For this review, take the finished solid that the model builds, in its own axes (mm). A direction names the side the tool comes from. Coordinates: 2 decimals unless noted, no trailing zeros. Write each loop counter-clockwise with the first axis right and the second up, starting at its lowest first coordinate (ties: lowest second). Pieces come first, ordered by that corner, then holes. Notation, with made-up numbers: M 8,76 L 25,76 A12 cw 25,91 Z; hole C -6,63 d9. An arc over 180 degrees is marked long. Return JSON: item names as keys, results as strings.
```python
from build123d import *

# Parameters (mm, degrees)
SKETCH2_R            = 9.9
BOSS_EXTRUDE1_DEPTH  = 1.225
SKETCH3_R            = 4.5
BOSS_EXTRUDE2_DEPTH  = 2.05
M3_CLEARANCE_HOLE1_D = 3.4


with BuildPart() as part:
    # Sketch2 → Boss-Extrude1 (new body, symmetric)
    with BuildSketch(Plane(origin=(0, 0, 0), x_dir=(1, 0, 0), z_dir=(0, 1, 0))):
        Circle(SKETCH2_R)
    extrude(amount=BOSS_EXTRUDE1_DEPTH, both=True)

    # Sketch3 → Boss-Extrude2 (add)
    with BuildSketch(Plane(origin=(0, 1.225, 0), x_dir=(1, 0, 0), z_dir=(0, 1, 0))):
        Circle(SKETCH3_R)
    extrude(amount=BOSS_EXTRUDE2_DEPTH)

    # M3 Clearance Hole1 (through all)
    with Locations(Plane(origin=(0, -1.225, 0), x_dir=(-1, 0, 0), z_dir=(0, -1, 0))):
        with Locations((0, 0), (0, 7), (7, 0), (0, -7), (-7, 0)):
            Hole(M3_CLEARANCE_HOLE1_D / 2)


solid = part.part
```
1. We need section C-C (x = 6). State the section outline as (y, z) points (3 decimals).
Checks:
{"outline": "M -1.225,-7.875 L 1.225,-7.875 L 1.225,-1.375 L -1.225,-1.375 Z; M -1.225,1.375 L 1.225,1.375 L 1.225,7.875 L -1.225,7.875 Z"}
2. Clearance check with flat-ended pins moving along their axes: pin 1 Ø1 at (y, z) = (1.5, 6.5) entering from +X; pin 2 Ø1.5 at (x, y) = (3, 1) entering from +Z; pin 3 Ø1 at (x, z) = (-6.5, -5) entering from +Y (3 decimals). State where each tip first meets the part, or that it passes through.
Checks:
{"pin 1": "x = 7.81", "pin 2": "z = 9.64", "pin 3": "y = 1.225"}
3. We need section A-A (z = 0). State the section outline as (x, y) points (3 decimals), plus the area to 3 significant figures.
Checks:
{"outline": "M -9.9,-1.225 L -8.7,-1.225 L -8.7,1.225 L -9.9,1.225 Z; M -5.3,-1.225 L -1.7,-1.225 L -1.7,3.275 L -4.5,3.275 L -4.5,1.225 L -5.3,1.225 Z; M 1.7,-1.225 L 5.3,-1.225 L 5.3,1.225 L 4.5,1.225 L 4.5,3.275 L 1.7,3.275 Z; M 8.7,-1.225 L 9.9,-1.225 L 9.9,1.225 L 8.7,1.225 Z", "area": "35.0 mm2"}
4. We need section B-B (x = 0). State the section outline as (y, z) points (3 decimals).
Checks:
{"outline": "M -1.225,-9.9 L 1.225,-9.9 L 1.225,-8.7 L -1.225,-8.7 Z; M -1.225,-5.3 L 1.225,-5.3 L 1.225,-4.5 L 3.275,-4.5 L 3.275,-1.7 L -1.225,-1.7 Z; M -1.225,1.7 L 3.275,1.7 L 3.275,4.5 L 1.225,4.5 L 1.225,5.3 L -1.225,5.3 Z; M -1.225,8.7 L 1.225,8.7 L 1.225,9.9 L -1.225,9.9 Z"}
5. We need section D-D (y = -0.85). State the section outline as (x, z) points, plus the area to 3 significant figures.
Checks:
{"outline": "C 0,0 d19.8; hole C -7,0 d3.4; hole C 0,-7 d3.4; hole C 0,0 d3.4; hole C 0,7 d3.4; hole C 7,0 d3.4", "area": "263 mm2"}
6. For faces 4 (the face through (-8.35, 0.02, 1.03)), 5 (the face through (-5, 1.225, 0)), list the 3-axis set-ups (+Z, -Z, +X, -X, +Y, -Y) from which the entire face can be reached by the end or side of a thin tool; tool diameter is ignored.
Checks:
{"face 4": "+Y, -Y", "face 5": "+Y"}
7. Wall thickness on L1, parallel to Z at x = 0, y = -0.55; L2, parallel to Y at x = 4, z = 8.75 (3 decimals); L3, parallel to X at y = 0, z = -7: over which ranges is each line inside the solid? List them lowest first. Write a range as from..to.
Checks:
{"L1": "-9.9..-8.7, -5.3..-1.7, 1.7..5.3, 8.7..9.9", "L2": "-1.225..1.225", "L3": "-7..-1.7, 1.7..7"}
8. Draft analysis for pull direction X (two halves, no side actions). For faces 1 (the face through (0, -1.225, 2)), 2 (the face through (5.65, 0.02, 1.03)), 3 (the face through (-0.59, 2.24, -4.46)), state which applies: +X half, -X half, draft (parallel to the pull), parting line (faces both ways), or undercut.
Checks:
{"face 1": "draft", "face 2": "undercut", "face 3": "parting line"}
